Can you work these out from the model? Positions are in its coordinate system, mm. Round coordinates to 2 decimals unless told otherwise and drop trailing zeros. Loops run counter-clockwise (first coordinate to the right, second up) from the corner with the lowest first, then second, coordinate; pieces in that order, holes last.
```python
from build123d import *

# Parameters (mm, degrees)
F1_DEPTH = 19.05
F2_W     = 152.4
F2_H     = 19.304
F3_DEPTH = 19.051
F4_W     = 6.35
F4_H     = 6.35
F5_DEPTH = 609.601


with BuildPart() as f1:
    # F0 (on Top) → F1 (new body)
    with BuildSketch(Plane.XY):
        Polygon((-158.75611, 188.8015), (-234.95611, 188.8015), (-234.95611, 87.67615), (-215.90611, 87.67615), (-215.90611, -13.92385), (-234.95611, -13.92385), (-234.95611, -115.9985), (-158.75611, -115.9985), (-158.75611, -96.9485), (-6.35611, -96.9485), (-6.35611, -115.9985), (146.04389, -115.9985), (146.04389, -96.9485), (298.44389, -96.9485), (298.44389, -115.9985), (374.64389, -115.9985), (374.64389, -14.3985), (355.59389, -14.3985), (355.59389, 87.2015), (374.64389, 87.2015), (374.64389, 188.8015), (298.44389, 188.8015), align=None)
    extrude(amount=F1_DEPTH)

    # F2 (on face) → F3 (cut, through all)
    with BuildSketch(Plane.XY.offset(19.05)):
        with Locations((-82.55611, 36.87615)):
            Rectangle(F2_W, F2_H)
        with Locations((222.24389, 36.87615)):
            Rectangle(F2_W, F2_H)
    extrude(amount=-F3_DEPTH, mode=Mode.SUBTRACT)

    # F4 (on face) → F5 (cut, through all)
    with BuildSketch(Plane.YZ.offset(374.64389)):
        with Locations((166.5765, 15.875)):
            Rectangle(F4_W, F4_H)
    extrude(amount=-F5_DEPTH, mode=Mode.SUBTRACT)


solid = f1.part
```
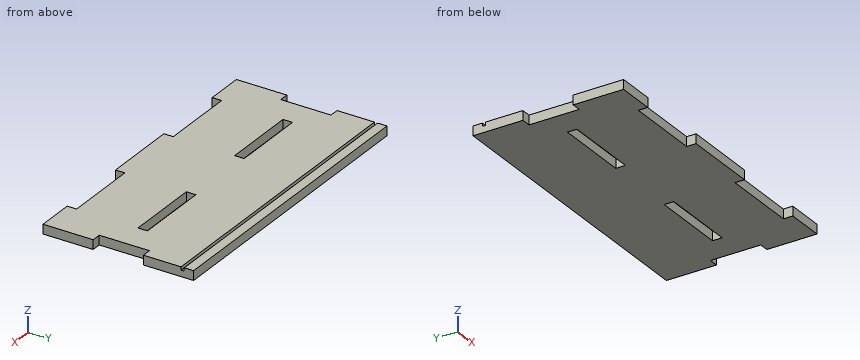
(1) For pin 1 (1 mm diameter, centred on x = 85.5, y = -46.5, fed in from -Z); pin 2 (5.5 mm diameter, centred on y = 35.5, z = 7.5, fed in from -X); pin 3 (9.5 mm diameter, centred on y = 58, z = 13, fed in from +X); pin 4 (5 mm diameter, centred on x = -49.5, z = 6.5, fed in from -Y), each with a flat end and sliding along its axis, tell me the tip position at first contact or that it passes through.
(2) If I drill on line 1 (X direction, y = 29, z = 8.25); line 2 (Y direction, x = 282, z = 15); line 3 (Y direction, x = -153.5, z = 4), over which ranges is the centre line in solid material (lowest first)?
(3) Suppose I cut it at C-C (y = 58). Write out the boundary of the cut face in (x, z).
(4) Suppose I cut it at A-A (z = 15.75). Give the number of separate pieces and of enclosed holes in the cut face, then the cut area to 3 significant figures.
(5) Suppose I cut it at B-B (x = 162.5). Write out the boundary of the cut face in (y, z), then the cut area to 3 significant figures.
Check result:
1. pin 1: stops at z = 0
1. pin 2: stops at x = -215.91
1. pin 3: stops at x = 355.59
1. pin 4: stops at y = -96.95
2. line 1: x = -215.91 to -158.76, -6.36 to 146.04, 298.44 to 355.59
2. line 2: y = -96.95 to 27.22, 46.53 to 163.4, 169.75 to 188.8
2. line 3: y = -96.95 to 27.22, 46.53 to 188.8
3. outline: (-215.91, 0) - (355.59, 0) - (355.59, 19.05) - (-215.91, 19.05) - close
4. separate pieces: 2
4. enclosed holes: 2
4. area: 166,000 mm2
5. outline: (-96.95, 0) - (27.22, 0) - (27.22, 19.05) - (-96.95, 19.05) - close; (46.53, 0) - (188.8, 0) - (188.8, 19.05) - (169.75, 19.05) - (169.75, 12.7) - (163.4, 12.7) - (163.4, 19.05) - (46.53, 19.05) - close
5. area: 5,040 mm2
